```python
from build123d import *

# Parameters (mm, degrees)
SKETCH_1_W      = 45
SKETCH_1_H      = 50.1
SKETCH_1_R      = 1.5
SKETCH_1_W_2    = 34.330352234
SKETCH_1_H_2    = 30.1
EXTRUDE_1_DEPTH = 3
FILLET_1_R      = 5


with BuildPart() as part:
    # 草图1 → 凸台-拉伸1 (new body)
    with BuildSketch(Plane.XY):
        with Locations((22.5, 25.05)):
            Rectangle(SKETCH_1_W, SKETCH_1_H)
        with Locations((10.5, 46.1)):
            Circle(SKETCH_1_R, mode=Mode.SUBTRACT)
        with Locations((34.5, 46.1)):
            Circle(SKETCH_1_R, mode=Mode.SUBTRACT)
        with Locations(Location((34.5, 4, 0), (0, 0, 180))):
            Circle(SKETCH_1_R, mode=Mode.SUBTRACT)
        with Locations(Location((10.5, 4, 0), (0, 0, 180))):
            Circle(SKETCH_1_R, mode=Mode.SUBTRACT)
        with Locations((22.5, 25.05)):
            Rectangle(SKETCH_1_W_2, SKETCH_1_H_2, mode=Mode.SUBTRACT)
    extrude(amount=EXTRUDE_1_DEPTH)

    # 圆角1
    fillet_1_edges = [part.edges().sort_by_distance(p)[0] for p in [
        (0, 50.1, 1.5),
        (45, 50.1, 1.5),
        (45, 0, 1.5),
        (0, 0, 1.5),
    ]]
    fillet(fillet_1_edges, radius=FILLET_1_R)


solid = part.part
```
Input: part model. Units: mm. Frame: model coordinates. A direction names the side the tool comes from. Give positions to 0.01 mm unless a question says otherwise; leave off trailing zeros. Order: outer loops, then holes, each group sorted by start corner. A loop starts at its lowest first (then second) coordinate and runs counter-clockwise, first axis right, second up. Notation, with made-up numbers: M 84.5,-20.75 L 122.5,-20.75 A20 cw 122.5,1.25 Z; hole C 66.25,80 d1. An arc over 180 degrees is marked long. Return JSON: item names as keys, results as strings.
1) Section query C-C on y = 23.5. Output: boundary loops of the cut face in (x, z), and give its area (3 significant figures).
Taken from the geometry:
{"outline": "M 0,0 L 5.33,0 L 5.33,3 L 0,3 Z; M 39.67,0 L 45,0 L 45,3 L 39.67,3 Z", "area": "32.0 mm2"}
2) Contact query for a flat-ended pin moving along its axis: pin 1 (3.5 mm diameter, centred on x = 34.5, y = 46.1, fed in from +Z). Output: stop coordinate, or through.
Taken from the geometry:
{"pin 1": "stops at z = 3"}
3) Section query D-D on z = 2.4. Output: boundary loops of the cut face in (x, y).
Taken from the geometry:
{"outline": "M 0,5 A5 ccw 5,0 L 40,0 A5 ccw 45,5 L 45,45.1 A5 ccw 40,50.1 L 5,50.1 A5 ccw 0,45.1 Z; hole M 5.33,10 L 39.67,10 L 39.67,40.1 L 5.33,40.1 Z; hole C 10.5,4 d3; hole C 10.5,46.1 d3; hole C 34.5,4 d3; hole C 34.5,46.1 d3"}
4) Mould query, pull axis Y, two halves, no side actions, for faces 3 (the face through (22, 0, 1)), 4 (the face through (22, 10, 1)), 5 (the face through (0, 25, 1)). Classes: released by +Y, released by -Y, zero draft, split by the parting line, or undercut.
Taken from the geometry:
{"face 3": "released by -Y", "face 4": "undercut", "face 5": "zero draft"}
5) Section query A-A on x = 22.5. Output: boundary loops of the cut face in (y, z), and give its area (3 significant figures).
Taken from the geometry:
{"outline": "M 0,0 L 10,0 L 10,3 L 0,3 Z; M 40.1,0 L 50.1,0 L 50.1,3 L 40.1,3 Z", "area": "60.0 mm2"}
6) Line query: L1, parallel to Y at x = 34.5, z = 2.15; L2, parallel to X at y = 18, z = 1.1; L3, parallel to Y at x = 24, z = 0.3. Output: solid intervals per line, ascending. Write a range as [from, to].
Taken from the geometry:
{"L1": "y = [0, 2.5], [5.5, 10], [40.1, 44.6], [47.6, 50.1]", "L2": "x = [0, 5.33], [39.67, 45]", "L3": "y = [0, 10], [40.1, 50.1]"}
7) Access query for faces 1 (the face through (43, 1, 2)), 2 (the face through (39.665, 25, 1)). Directions: +Z, -Z, +X, -X, +Y, -Y. A direction counts if a zero-diameter tool reaches every point of the face in a straight line with its end or side. Return the directions, or none.
Taken from the geometry:
{"face 1": "+Z, -Z, +X, -Y", "face 2": "+Z, -Z"}
8) Section query B-B on x = 10.5. Output: boundary loops of the cut face in (y, z), and give its area (3 significant figures).
Taken from the geometry:
{"outline": "M 0,0 L 2.5,0 L 2.5,3 L 0,3 Z; M 5.5,0 L 10,0 L 10,3 L 5.5,3 Z; M 40.1,0 L 44.6,0 L 44.6,3 L 40.1,3 Z; M 47.6,0 L 50.1,0 L 50.1,3 L 47.6,3 Z", "area": "42.0 mm2"}
